Source: three-view drawing plus pictorial views. Frame: mm from the lowest corner of the part. Round coordinates to 2 decimals unless told otherwise and drop trailing zeros. Loops run counter-clockwise (first coordinate to the right, second up) from the corner with the lowest first, then second, coordinate; pieces in that order, holes last. Notation, with made-up numbers: (-30, 21) -> (-9, 21) arc R36 ccw to (-9, 59) -> close; hole circle Ø1 at (-5, -33.75). An arc over 180 degrees is marked (long way). Put each result on its own line as item: value. Start each with the question number.
1. Cut plane A-A (z = 28.75). Return the cut outline in (x, y), then the cut area to 3 significant figures.
2. Material intervals for L1, parallel to X at y = 3.75, z = 28.75; L2, parallel to Z at x = 16.5, y = 11.25, sorted ascending.
3. Cut plane B-B (x = 16.5). Return the cut outline in (y, z), then the cut area to 3 significant figures.
4. Contact query for flat-ended pins moving along their axis: pin 1 (6.5 mm diameter, centred on x = 16.5, z = 28.75, fed in from +Y); pin 2 (3 mm diameter, centred on x = 73.75, z = 28.75, fed in from -Y). Output: stop coordinate, or through.
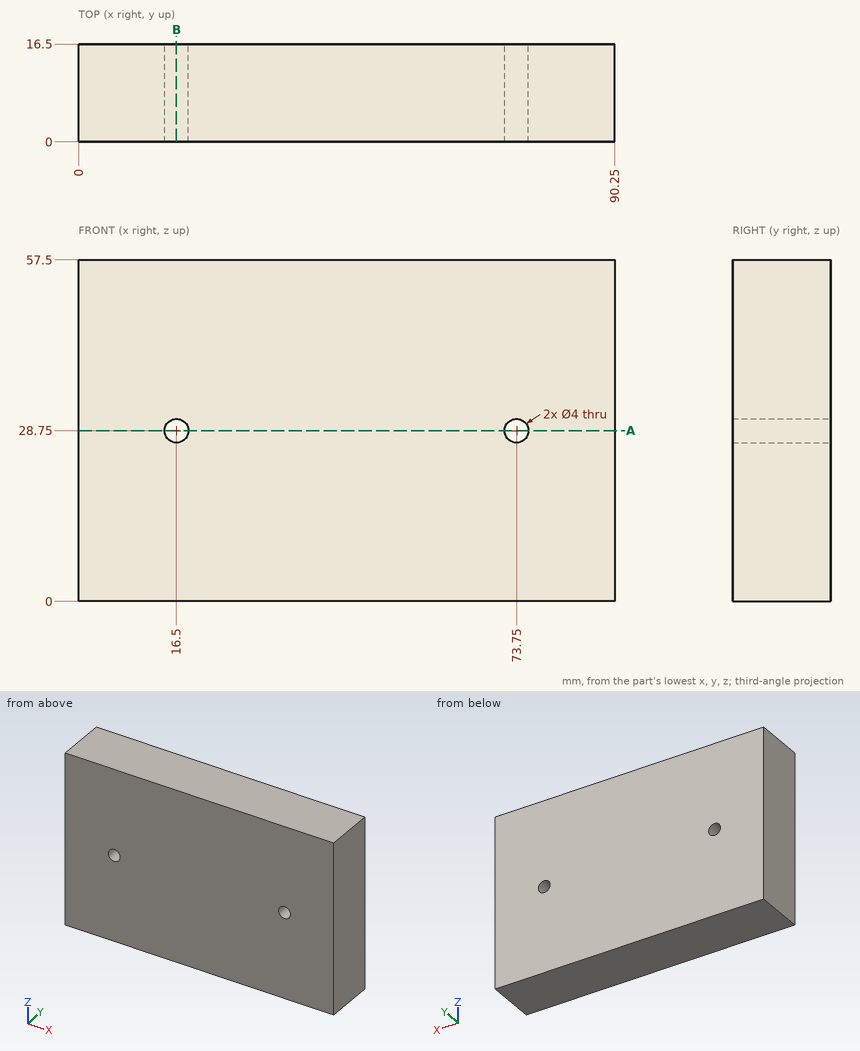
Solution:
1. outline: (0, 0) -> (14.5, 0) -> (14.5, 16.5) -> (0, 16.5) -> close; (18.5, 0) -> (71.75, 0) -> (71.75, 16.5) -> (18.5, 16.5) -> close; (75.75, 0) -> (90.25, 0) -> (90.25, 16.5) -> (75.75, 16.5) -> close
1. area: 1,360 mm^2
2. L1: x = 0 to 14.5, 18.5 to 71.75, 75.75 to 90.25
2. L2: z = 0 to 26.75, 30.75 to 57.5
3. outline: (0, 0) -> (16.5, 0) -> (16.5, 26.75) -> (0, 26.75) -> close; (0, 30.75) -> (16.5, 30.75) -> (16.5, 57.5) -> (0, 57.5) -> close
3. area: 883 mm^2
4. pin 1: stops at y = 16.5
4. pin 2: passes through
